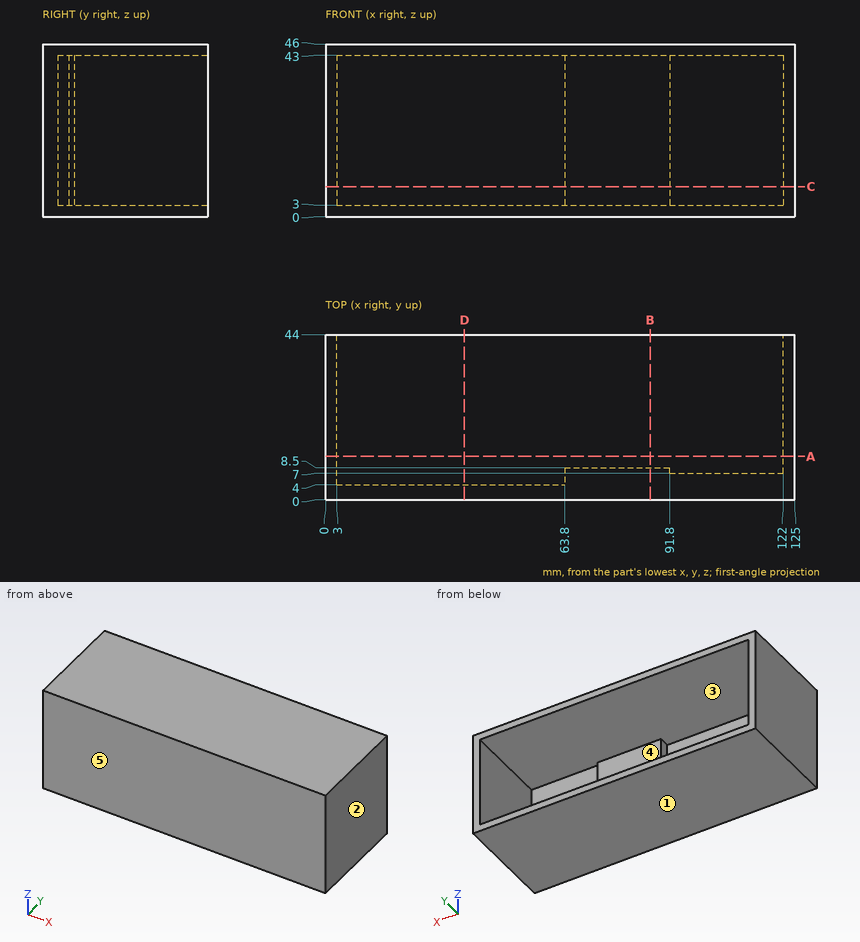
Drawing for the job (mm, zero at the part's lowest x, y, z). A direction names the side the tool comes from. Round coordinates to 2 decimals unless told otherwise and drop trailing zeros. Write each loop counter-clockwise with the first axis right and the second up, starting at its lowest first coordinate (ties: lowest second). Pieces come first, ordered by that corner, then holes. Notation, with made-up numbers: M -5,-30 L 13,-30 A21 ccw 13,-6 Z; hole C 89.25,13 d11. An arc over 180 degrees is marked long. Answer as a JSON object with one key per item and string values. Group by question number.
(1) Which spindle directions (+Z, -Z, +X, -X, +Y, -Y) get a long thin tool onto all of the face, cutting with end or side? Do the marked faces 4 and 5. Say none if no direction does.
(2) Mould opens along X. For the marked faces 1, 2 and 3 say: pulls with the +X half, pulls with the -X half, needs draft (parallel to the pull), parting line crosses it, or undercut.
(3) Drill centre lines: L1, parallel to Z at x = 84.5, y = 40.5; L2, parallel to X at y = 16, z = 25; L3, parallel to X at y = 7.5, z = 16. Where is each one in solid material? Low to high.
(4) Cut at D-D (x = 37). Give the cut face in (y, z), and give its area (3 significant figures).
(5) Cut at B-B (x = 86.5). Give the cut face in (y, z).
(6) Cut at C-C (z = 8). Give the cut face in (x, y).
(7) Cut at A-A (y = 11.5). Give the cut face in (x, z).
(8) Flat gauge pins, fed straight in: pin 1 (15 mm diameter, centred on x = 105.5, z = 26, fed in from +Y); pin 2 (4 mm diameter, centred on x = 23.5, z = 21, fed in from +Y); pin 3 (22.5 mm diameter, centred on x = 76, z = 16, fed in from +Y). Where does each tip first touch, or does it go through?
Responses:
{
 "1": {"face 4": "+Y", "face 5": "+Z, -Z, +X, -X, -Y"},
 "2": {"face 1": "needs draft", "face 2": "pulls with the +X half", "face 3": "undercut"},
 "3": {"L1": "z = 0 to 3, 43 to 46", "L2": "x = 0 to 3, 122 to 125", "L3": "x = 0 to 3, 63.8 to 91.8, 122 to 125"},
 "4": {"outline": "M 0,0 L 44,0 L 44,3 L 4,3 L 4,43 L 44,43 L 44,46 L 0,46 Z", "area": "424 mm2"},
 "5": {"outline": "M 0,0 L 44,0 L 44,3 L 8.5,3 L 8.5,43 L 44,43 L 44,46 L 0,46 Z"},
 "6": {"outline": "M 0,0 L 125,0 L 125,44 L 122,44 L 122,7 L 91.8,7 L 91.8,8.5 L 63.8,8.5 L 63.8,4 L 3,4 L 3,44 L 0,44 Z"},
 "7": {"outline": "M 0,0 L 125,0 L 125,46 L 0,46 Z; hole M 3,3 L 122,3 L 122,43 L 3,43 Z"},
 "8": {"pin 1": "stops at y = 7", "pin 2": "stops at y = 4", "pin 3": "stops at y = 8.5"}
}
